Here's how the part is built. I have some questions about the finished solid (model axes, mm). Face numbers are marked on the shaded views. A direction names the side the tool comes from. Give positions to 0.01 mm unless a question says otherwise; leave off trailing zeros. Order: outer loops, then holes, each group sorted by start corner. A loop starts at its lowest first (then second) coordinate and runs counter-clockwise, first axis right, second up.
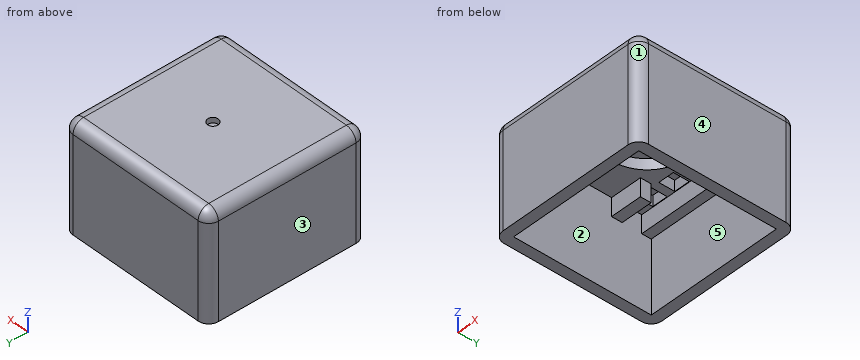
from build123d import *

# Parameters (mm, degrees)
CYLINDER002_R     = 1
CYLINDER002_DEPTH = 1
BOX006_W          = 3
BOX006_H          = 3
BOX006_DEPTH      = 2
BOX005_W          = 3
BOX005_H          = 3
BOX005_DEPTH      = 2
BOX003_W          = 3
BOX003_H          = 3
BOX003_DEPTH      = 2
BOX004_W          = 3
BOX004_H          = 3
BOX004_DEPTH      = 2
BOX002_W          = 3
BOX002_H          = 3
BOX002_DEPTH      = 2
CYLINDER_R        = 7
CYLINDER_DEPTH    = 2
BOX_W             = 26
BOX_H             = 26
BOX_DEPTH         = 17
BOX001_W          = 30
BOX001_H          = 30
BOX001_DEPTH      = 20
CYLINDER001_R     = 3
CYLINDER001_DEPTH = 2
BOX010_W          = 6
BOX010_H          = 2
BOX010_DEPTH      = 3.4
BOX008_W          = 4
BOX008_H          = 4
BOX008_DEPTH      = 3.4
BOX007_W          = 26
BOX007_H          = 1.8
BOX007_DEPTH      = 3.4
BOX009_W          = 6
BOX009_H          = 2
BOX009_DEPTH      = 3.4
BOX011_W          = 6
BOX011_H          = 2
BOX011_DEPTH      = 3.4
FILLET_R          = 2


with BuildPart() as obj1:
    # Cylinder002 → Cylinder002 (new body)
    with BuildSketch(Plane(origin=(0.1, 0.3, 9), x_dir=(1, 0, 0), z_dir=(0, 0, 1))):
        Circle(CYLINDER002_R)
    extrude(amount=CYLINDER002_DEPTH)


with BuildPart() as l5:
    # Box006 → Box006 (new body)
    with BuildSketch(Plane(origin=(7.67, 8.11, 7), x_dir=(1, 0, 0), z_dir=(0, 0, 1))):
        with Locations((1.5, 1.5)):
            Rectangle(BOX006_W, BOX006_H)
    extrude(amount=BOX006_DEPTH)


with BuildPart() as l4:
    # Box005 → Box005 (new body)
    with BuildSketch(Plane(origin=(3.1, 8.11, 7), x_dir=(1, 0, 0), z_dir=(0, 0, 1))):
        with Locations((1.5, 1.5)):
            Rectangle(BOX005_W, BOX005_H)
    extrude(amount=BOX005_DEPTH)


with BuildPart() as l2:
    # Box003 → Box003 (new body)
    with BuildSketch(Plane(origin=(-6.04, 8.11, 7), x_dir=(1, 0, 0), z_dir=(0, 0, 1))):
        with Locations((1.5, 1.5)):
            Rectangle(BOX003_W, BOX003_H)
    extrude(amount=BOX003_DEPTH)


with BuildPart() as l3:
    # Box004 → Box004 (new body)
    with BuildSketch(Plane(origin=(-1.47, 8.11, 7), x_dir=(1, 0, 0), z_dir=(0, 0, 1))):
        with Locations((1.5, 1.5)):
            Rectangle(BOX004_W, BOX004_H)
    extrude(amount=BOX004_DEPTH)


with BuildPart() as fusion:
    # Box002 → Box002 (new body)
    with BuildSketch(Plane(origin=(-10.61, 8.11, 7), x_dir=(1, 0, 0), z_dir=(0, 0, 1))):
        with Locations((1.5, 1.5)):
            Rectangle(BOX002_W, BOX002_H)
    extrude(amount=BOX002_DEPTH)

    # Fusion: union L5, L4, L2, L3
    add(l5.part)
    add(l4.part)
    add(l2.part)
    add(l3.part)


with BuildPart() as but:
    # Cylinder → Cylinder (new body)
    with BuildSketch(Plane(origin=(0.1, 0.3, 7), x_dir=(1, 0, 0), z_dir=(0, 0, 1))):
        Circle(CYLINDER_R)
    extrude(amount=CYLINDER_DEPTH)


with BuildPart() as maininside:
    # Box → Box (new body)
    with BuildSketch(Plane(origin=(-13, -13, -10), x_dir=(1, 0, 0), z_dir=(0, 0, 1))):
        with Locations((13, 13)):
            Rectangle(BOX_W, BOX_H)
    extrude(amount=BOX_DEPTH)


with BuildPart() as cut002:
    # Box001 → Box001 (new body)
    with BuildSketch(Plane(origin=(-15, -15, -10), x_dir=(1, 0, 0), z_dir=(0, 0, 1))):
        with Locations((15, 15)):
            Rectangle(BOX001_W, BOX001_H)
    extrude(amount=BOX001_DEPTH)

    # Cut: cut MainInside
    add(maininside.part, mode=Mode.SUBTRACT)

    # Cut001: cut But
    add(but.part, mode=Mode.SUBTRACT)

    # Cut002: cut Fusion
    add(fusion.part, mode=Mode.SUBTRACT)


with BuildPart() as cut003:
    # Cylinder001 → Cylinder001 (new body)
    with BuildSketch(Plane(origin=(0.1, 0.3, 8), x_dir=(1, 0, 0), z_dir=(0, 0, 1))):
        Circle(CYLINDER001_R)
    extrude(amount=CYLINDER001_DEPTH)

    # Fusion001: union Cut002
    add(cut002.part)

    # Cut003: cut obj1
    add(obj1.part, mode=Mode.SUBTRACT)


with BuildPart() as obj2:
    # Box010 → Box010 (new body)
    with BuildSketch(Plane(origin=(-13, 5.5, 3.6), x_dir=(1, 0, 0), z_dir=(0, 0, 1))):
        with Locations((3, 1)):
            Rectangle(BOX010_W, BOX010_H)
    extrude(amount=BOX010_DEPTH)


with BuildPart() as obj3:
    # Box008 → Box008 (new body)
    with BuildSketch(Plane(origin=(8, 0, 3.6), x_dir=(1, 0, 0), z_dir=(0, 0, 1))):
        with Locations((2, 2)):
            Rectangle(BOX008_W, BOX008_H)
    extrude(amount=BOX008_DEPTH)


with BuildPart() as obj4:
    # Box007 → Box007 (new body)
    with BuildSketch(Plane(origin=(-13, 11.2, 3.6), x_dir=(1, 0, 0), z_dir=(0, 0, 1))):
        with Locations((13, 0.9)):
            Rectangle(BOX007_W, BOX007_H)
    extrude(amount=BOX007_DEPTH)


with BuildPart() as obj5:
    # Box009 → Box009 (new body)
    with BuildSketch(Plane(origin=(-13, -4, 3.6), x_dir=(1, 0, 0), z_dir=(0, 0, 1))):
        with Locations((3, 1)):
            Rectangle(BOX009_W, BOX009_H)
    extrude(amount=BOX009_DEPTH)


with BuildPart() as fillet_body:
    # Box011 → Box011 (new body)
    with BuildSketch(Plane(origin=(7, -13, 3.6), x_dir=(1, 0, 0), z_dir=(0, 0, 1))):
        with Locations((3, 1)):
            Rectangle(BOX011_W, BOX011_H)
    extrude(amount=BOX011_DEPTH)

    # Fusion002: union obj2, obj3, obj4, obj5
    add(obj2.part)
    add(obj3.part)
    add(obj4.part)
    add(obj5.part)

    # Fusion003: union Cut003
    add(cut003.part)

    # Fillet
    fillet_edges = [fillet_body.edges().sort_by_distance(p)[0] for p in [
        (-15, -15, 0),
        (-15, 0, 10),
        (-15, 15, 0),
        (15, 15, 0),
        (0, 15, 10),
        (15, -15, 0),
        (0, -15, 10),
        (15, 0, 10),
    ]]
    fillet(fillet_edges, radius=FILLET_R)


solid = fillet_body.part
Q1. For the marked faces 4 and 5, which set-ups out of +Z, -Z, +X, -X, +Y, -Y let a thin tool reach every point of the face, with its end or its side?
Filled sheet:
face 4: +Z, -Z, +X, +Y, -Y
face 5: -Z
Q2. If we section it at B-B on z = 1.25: List the corners of the cut face in (x, y) for me.
Filled sheet:
outline: (-15, -13) arc R2 ccw to (-13, -15) - (13, -15) arc R2 ccw to (15, -13) - (15, 13) arc R2 ccw to (13, 15) - (-13, 15) arc R2 ccw to (-15, 13) - close; hole (-13, -13) - (13, -13) - (13, 13) - (-13, 13) - close
Q3. Thinking about a two-plate mould opening in Y: for the marked faces 1, 2 and 3, which applies, released by +Y, released by -Y, zero draft, split by the parting line, or undercut?
Filled sheet:
face 1: released by -Y
face 2: undercut
face 3: zero draft
Q4. If we section it at D-D on z = 8.5: Give the number of separate pieces and of enclosed holes in the cut face, plus the area to 3 significant figures.
Filled sheet:
separate pieces: 2
enclosed holes: 6
area: 719 mm2
Q5. I'm going to push flat-ended pins straight in: P1, Ø1, axis at x = 1, y = 7.5, coming from the -Z side; P2, Ø3.5, axis at x = -9, y = 10, coming from the -Z side; P3, Ø1.6, axis at x = -0.5, z = 8.5, coming from the -Y side; P4, Ø1.8, axis at x = 0.1, y = 0.3, coming from the -Z side. Where does each tip first touch, or does it pass through?
Filled sheet:
P1: stops at z = 7
P2: stops at z = 3.6
P3: stops at y = -15
P4: stops at z = 8
Q6. If we section it at A-A on z = 6: List the corners of the cut face in (x, y) for me.
Filled sheet:
outline: (-15, -13) arc R2 ccw to (-13, -15) - (13, -15) arc R2 ccw to (15, -13) - (15, 13) arc R2 ccw to (13, 15) - (-13, 15) arc R2 ccw to (-15, 13) - close; (8, 0) - (12, 0) - (12, 4) - (8, 4) - close; hole (-13, -13) - (7, -13) - (7, -11) - (13, -11) - (13, 11.2) - (-13, 11.2) - (-13, 7.5) - (-7, 7.5) - (-7, 5.5) - (-13, 5.5) - (-13, -2) - (-7, -2) - (-7, -4) - (-13, -4) - close
Q7. I need wall thicknesses on L1, parallel to X at y = 8, z = 6.25; L2, parallel to Y at x = -12.5, z = 6. Which ranges of each line are inside material? Lowest first, please.
Filled sheet:
L1: x = -15 to -13, 13 to 15
L2: y = -15 to -13, -4 to -2, 5.5 to 7.5, 11.2 to 15
Q8. If we section it at C-C on x = 9: List the corners of the cut face in (y, z) for me.
Filled sheet:
outline: (-15, -10) - (-13, -10) - (-13, 3.6) - (-11, 3.6) - (-11, 7) - (0, 7) - (0, 3.6) - (4, 3.6) - (4, 7) - (8.11, 7) - (8.11, 9) - (11.11, 9) - (11.11, 7) - (11.2, 7) - (11.2, 3.6) - (13, 3.6) - (13, -10) - (15, -10) - (15, 8) arc R2 ccw to (13, 10) - (-13, 10) arc R2 ccw to (-15, 8) - close
